Geometry check sheet. Reference: the model listing, model coordinates, mm. Face numbers are marked on the shaded views. A direction names the side the tool comes from. Give positions to 0.01 mm unless a question says otherwise; leave off trailing zeros. Loops run counter-clockwise (first coordinate to the right, second up) from the corner with the lowest first, then second, coordinate; pieces in that order, holes last. Notation, with made-up numbers: (-33.75, 16) -> (22.25, 16) arc R25 cw to (22.25, 53) -> close; hole circle Ø1 at (44.5, 88). An arc over 180 degrees is marked (long way). Write item = value, one per line.
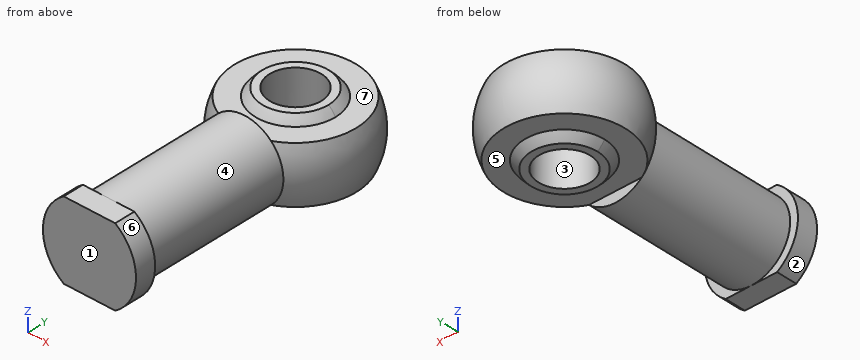
```python
from build123d import *
from build123d.topology import SkipClean

# Parameters (mm, degrees)
CUT_EXTRUDE3_DEPTH      = 59.940648113
CUT_EXTRUDE3_DEPTH_BACK = 59.940648113
SKETCH3_W               = 17.579289035
SKETCH3_H               = 30.509322749
CUT_EXTRUDE4_DEPTH      = 59.268773799
CUT_EXTRUDE4_DEPTH_BACK = 59.268773799
SKETCH4_W               = 14.932737824
SKETCH4_H               = 19.875765969
CUT_EXTRUDE5_DEPTH      = 60.674114991
CUT_EXTRUDE5_DEPTH_BACK = 60.674114991
SKETCH5_R               = 5
CUT_EXTRUDE6_DEPTH      = 59.189346104
CUT_EXTRUDE6_DEPTH_BACK = 59.189346104
SKETCH6_W               = 15.994671042
SKETCH6_H               = 5.292782054


with BuildPart() as part:
    # Sketch1 → Revolve5 (revolve)
    with SkipClean():  # the faces are left unmerged after this step: merging them gives an invalid solid
        with BuildSketch(Plane.XY, mode=Mode.PRIVATE) as revolve5_sk:
            with BuildLine():
                ThreePointArc((10.5, 43), (7.424621202, 50.424621202), (0, 53.5))
                Line((0, 53.5), (0, 52.5))
                ThreePointArc((0, 52.5), (6.717514421, 49.717514421), (9.5, 43))
                ThreePointArc((9.5, 43), (6.717514421, 36.282485579), (0, 33.5))
                Line((0, 33.5), (0, 32.5))
                ThreePointArc((0, 32.5), (7.424621202, 35.575378798), (10.5, 43))
            make_face()
            with BuildLine():
                Line((0, 52.5), (0, 53.5))
                ThreePointArc((0, 53.5), (-10.5, 43), (0, 32.5))
                Line((0, 32.5), (0, 33.5))
                ThreePointArc((0, 33.5), (-9.5, 43), (0, 52.5))
            make_face()
        revolve(revolve5_sk.sketch.rotate(Axis((0, 0, 0), (0, 1, 0)), 180), axis=Axis((0, 0, 0), (0, 1, 0)))

    # Sketch1_7 → Revolve6 (revolve)
    with SkipClean():  # the faces are left unmerged after this step: merging them gives an invalid solid
        with BuildSketch(Plane.XY, mode=Mode.PRIVATE) as revolve6_sk:
            with BuildLine():
                Line((-7.5, 32.381619709), (-7.5, 4))
                Line((-7.5, 4), (-9, 4))
                Line((-9, 4), (-9, 0))
                Line((-9, 0), (0, 0))
                Line((0, 0), (0, 30))
                ThreePointArc((0, 30), (-3.934530227, 30.60970251), (-7.5, 32.381619709))
            make_face()
            with BuildLine():
                ThreePointArc((0, 56), (-12.39029749, 46.934530227), (-7.5, 32.381619709))
                ThreePointArc((-7.5, 32.381619709), (-3.934530227, 30.60970251), (0, 30))
                Line((0, 30), (0, 32.5))
                ThreePointArc((0, 32.5), (-10.5, 43), (0, 53.5))
                Line((0, 53.5), (0, 56))
            make_face()
            with BuildLine():
                ThreePointArc((13, 43), (9.192388155, 52.192388155), (0, 56))
                Line((0, 56), (0, 53.5))
                ThreePointArc((0, 53.5), (7.424621202, 50.424621202), (10.5, 43))
                ThreePointArc((10.5, 43), (7.424621202, 35.575378798), (0, 32.5))
                Line((0, 32.5), (0, 30))
                ThreePointArc((0, 30), (9.192388155, 33.807611845), (13, 43))
            make_face()
        revolve(revolve6_sk.sketch.rotate(Axis((0, 0, 0), (0, 1, 0)), 270), axis=Axis((0, 0, 0), (0, 1, 0)))

    # Sketch3 → Cut-Extrude3 (cut, two sides: drawn at the far end of the back side and taken through both)
    with SkipClean():  # the faces are left unmerged after this step: merging them gives an invalid solid
        with BuildSketch(Plane(origin=(0, 0, 0), x_dir=(0, 0, -1), z_dir=(1, 0, 0)).offset(-CUT_EXTRUDE3_DEPTH_BACK)):
            with Locations((-14.289644518, 47.636281084)):
                Rectangle(SKETCH3_W, SKETCH3_H)
            with Locations((14.289644518, 47.636281084)):
                Rectangle(SKETCH3_W, SKETCH3_H)
        extrude(amount=CUT_EXTRUDE3_DEPTH + CUT_EXTRUDE3_DEPTH_BACK, mode=Mode.SUBTRACT)

    # Sketch1_8 → Revolve7 (revolve)
    with SkipClean():  # the faces are left unmerged after this step: merging them gives an invalid solid
        with BuildSketch(Plane.XY, mode=Mode.PRIVATE) as revolve7_sk:
            with BuildLine():
                ThreePointArc((9.5, 43), (6.717514421, 49.717514421), (0, 52.5))
                Line((0, 52.5), (0, 33.5))
                ThreePointArc((0, 33.5), (6.717514421, 36.282485579), (9.5, 43))
            make_face()
            with BuildLine():
                Line((0, 33.5), (0, 52.5))
                ThreePointArc((0, 52.5), (-9.5, 43), (0, 33.5))
            make_face()
        revolve(revolve7_sk.sketch.rotate(Axis((0, 0, 0), (0, 1, 0)), 180), axis=Axis((0, 0, 0), (0, 1, 0)))

    # Sketch4 → Cut-Extrude4 (cut, two sides: drawn at the far end of the back side and taken through both)
    with BuildSketch(Plane(origin=(0, 0, 0), x_dir=(0, 0, -1), z_dir=(1, 0, 0)).offset(-CUT_EXTRUDE4_DEPTH_BACK)):
        with Locations((-14.466368912, 45.402031304)):
            Rectangle(SKETCH4_W, SKETCH4_H)
        with Locations((14.466368912, 45.402031304)):
            Rectangle(SKETCH4_W, SKETCH4_H)
    extrude(amount=CUT_EXTRUDE4_DEPTH + CUT_EXTRUDE4_DEPTH_BACK, mode=Mode.SUBTRACT)

    # Sketch5 → Cut-Extrude5 (cut, two sides: drawn at the far end of the back side and taken through both)
    with BuildSketch(Plane.XY.offset(7).offset(-CUT_EXTRUDE5_DEPTH_BACK)):
        with Locations((0, 43)):
            Circle(SKETCH5_R)
    extrude(amount=CUT_EXTRUDE5_DEPTH + CUT_EXTRUDE5_DEPTH_BACK, mode=Mode.SUBTRACT)

    # Sketch6 → Cut-Extrude6 (cut, two sides: drawn at the far end of the back side and taken through both)
    with BuildSketch(Plane(origin=(0, 0, 0), x_dir=(1, 0, 0), z_dir=(0, 1, 0)).offset(-CUT_EXTRUDE6_DEPTH_BACK)):
        with Locations((0.436218301, 10.146391027)):
            Rectangle(SKETCH6_W, SKETCH6_H)
        with Locations((0.436218301, -10.146391027)):
            Rectangle(SKETCH6_W, SKETCH6_H)
    extrude(amount=CUT_EXTRUDE6_DEPTH + CUT_EXTRUDE6_DEPTH_BACK, mode=Mode.SUBTRACT)


solid = part.part
```
Item 1: Tool access check on the marked faces 4, 5, 6 and 7. Record the directions out of +Z, -Z, +X, -X, +Y, -Y that give a thin tool (end or side, any length) a straight path to the whole face; none if there is none.
Answer:
face_4 = none
face_5 = -Z
face_6 = +X, -Y
face_7 = +Z
Item 2: Section check B-B, the plane z = 4.75. Record the cut outline in (x, y).
Answer:
outline = (-7.64, 0) -> (7.64, 0) -> (7.64, 4) -> (5.8, 4) -> (5.8, 32.38) arc R12.1 ccw (long way) to (-5.8, 32.38) -> (-5.8, 4) -> (-7.64, 4) -> close; hole circle Ø10 at (0, 43)
Item 3: Section check A-A, the plane z = 0. Record the cut outline in (x, y), plus the area to 3 significant figures.
Answer:
outline = (-9, 0) -> (9, 0) -> (9, 4) -> (7.5, 4) -> (7.5, 32.38) arc R13 ccw (long way) to (-7.5, 32.38) -> (-7.5, 4) -> (-9, 4) -> close; hole circle Ø10 at (0, 43)
area = 926 mm^2
Item 4: Section check C-C, the plane y = 52.5. Record the cut outline in (x, z), plus the area to 3 significant figures.
Answer:
outline = (-6.96, -5.5) -> (6.96, -5.5) arc R8.87 ccw to (6.96, 5.5) -> (-6.96, 5.5) arc R8.87 ccw to start
area = 182 mm^2
Item 5: Draft check along Y on the marked faces 1, 2 and 3. Enter one of: +Y half, -Y half, draft (parallel to the pull), parting line (faces both ways), or undercut.
Answer:
face_1 = -Y half
face_2 = draft
face_3 = undercut
Item 6: Gauge pin test, flat ends, axial feed: pin 1 (6.5 mm diameter, centred on x = 2, y = 38.5, fed in from +Z); pin 2 (6.5 mm diameter, centred on x = -2.5, y = 47.5, fed in from -Z); pin 3 (1.6 mm diameter, centred on x = -0.5, z = 6.5, fed in from +Y). Record the tip position at first contact, or that the pin passes through.
Answer:
pin_1 = 7
pin_2 = -7
pin_3 = 50.59
Item 7: Thickness scan on L1, parallel to Y at x = 0, z = 0.25; L2, parallel to X at y = 43, z = -2.75; L3, parallel to Z at x = -2.25, y = 37. Record the ranges inside material, lowest first. Write a range as [from, to].
Answer:
L1 = [0, 38], [48, 56]
L2 = [-12.71, -5], [5, 12.71]
L3 = [-7, 7]
